Design review of the part shown in the three views and the two pictorial views. Dimensions are in mm from the part's minimum x, y and z. Give positions to 0.01 mm unless a question says otherwise; leave off trailing zeros. Write each loop counter-clockwise with the first axis right and the second up, starting at its lowest first coordinate (ties: lowest second). Pieces come first, ordered by that corner, then holes. Notation, with made-up numbers: M 28.25,-35 L 84.25,-35 A19 ccw 84.25,-7 Z; hole C 10.5,55 d9. An arc over 180 degrees is marked long. Write item = value, one per line.
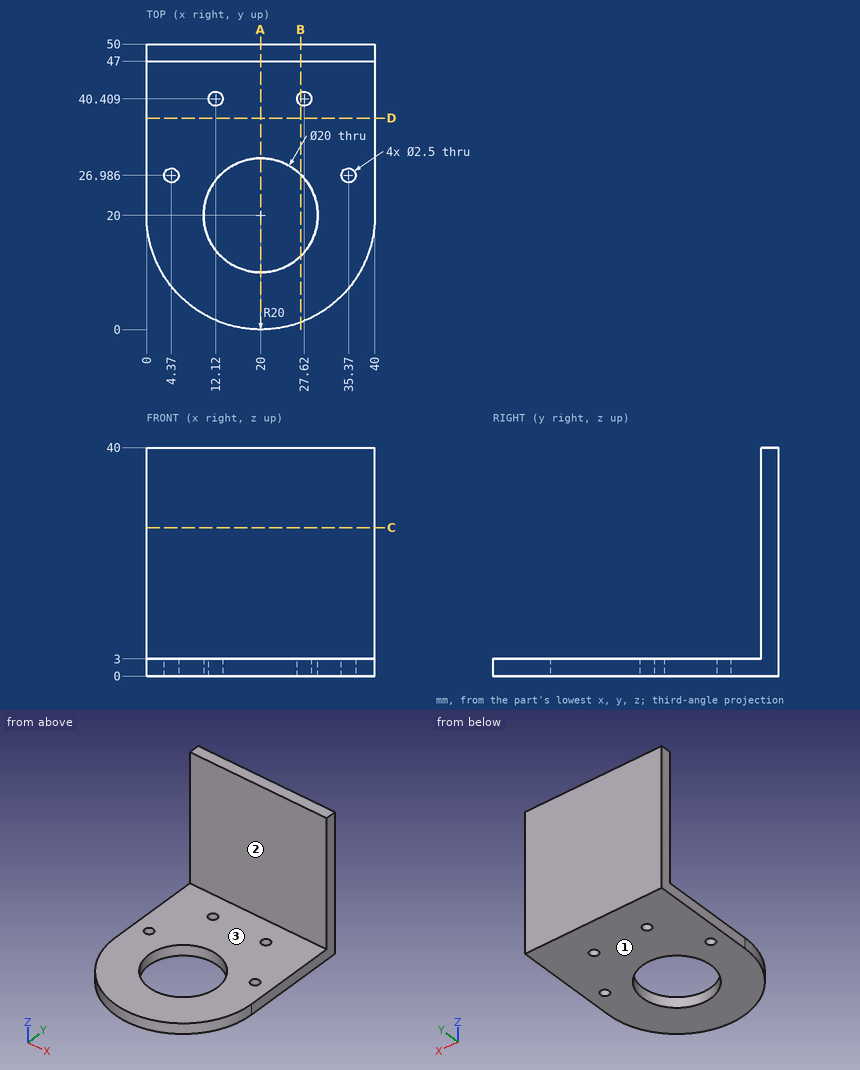
1. We need section B-B, the plane x = 27. Write out the cut boundary in (y, z) (1 decimal), then the cut area to 3 significant figures.
Responses:
outline = M 1.3,0 L 12.9,0 L 12.9,3 L 1.3,3 Z; M 27.1,0 L 39.3,0 L 39.3,3 L 27.1,3 Z; M 41.5,0 L 50,0 L 50,40 L 47,40 L 47,3 L 41.5,3 Z
area = 208 mm2
2. We need section A-A, the plane x = 20. Write out the cut boundary in (y, z).
Responses:
outline = M 0,0 L 10,0 L 10,3 L 0,3 Z; M 30,0 L 50,0 L 50,40 L 47,40 L 47,3 L 30,3 Z
3. For line 1 along Y through (x, z) = (20, 0.75); line 2 along Y through (x, z) = (14.5, 33); line 3 along Z through (x, y) = (36.5, 42), list the stretches that pass through material, from the lowest coordinate up. Write a range as from..to.
Responses:
line_1 = 0..10, 30..50
line_2 = 47..50
line_3 = 0..3
4. We need section D-D, the plane y = 37. Write out the cut boundary in (x, z), then the cut area to 3 significant figures.
Responses:
outline = M 0,0 L 40,0 L 40,3 L 0,3 Z
area = 120 mm2
5. Insertion check: P1, Ø2, axis at x = 4.37, y = 26.99, coming from the +Z side; P2, Ø6, axis at x = 8, z = 33, coming from the -Y side; P3, Ø3, axis at x = 12.12, y = 40.41, coming from the +Z side. Each pin has a flat end and moves straight along its axis. Give the tip position at first contact, or say it passes through.
Responses:
P1 = through
P2 = 47
P3 = 3
6. The part is to be moulded in two halves that separate along Z. For the marked faces 1, 2 and 3, say which applies: +Z half, -Z half, draft (parallel to the pull), parting line (faces both ways), or undercut.
Responses:
face_1 = -Z half
face_2 = draft
face_3 = +Z half
7. We need section C-C, the plane z = 26. Write out the cut boundary in (x, y), then the cut area to 3 significant figures.
Responses:
outline = M 0,47 L 40,47 L 40,50 L 0,50 Z
area = 120 mm2
